The drawing under review shows one solid part. Ordinate dimensions are in mm from its lowest x, y, z. Coordinates: 2 decimals unless noted, no trailing zeros. Write each loop counter-clockwise with the first axis right and the second up, starting at its lowest first coordinate (ties: lowest second). Pieces come first, ordered by that corner, then holes.
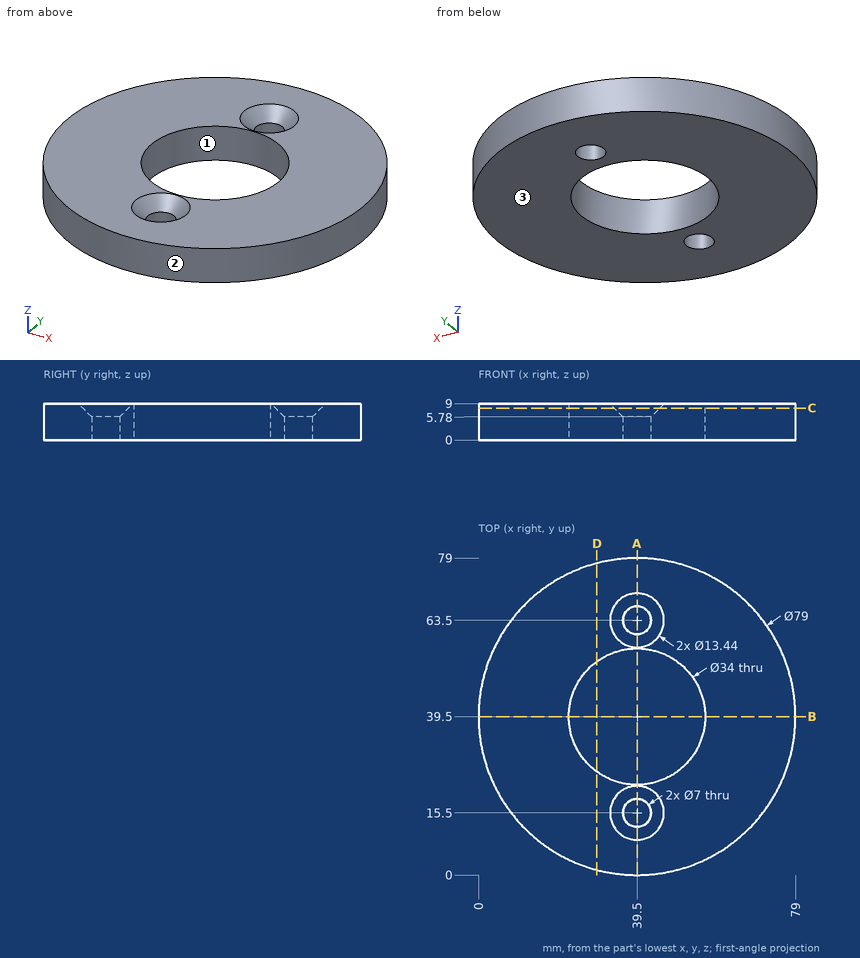
Q1. Add section B-B (y = 39.5). State the section outline as (x, z) points, then the cut area to 3 significant figures.
Ans:
outline: (0, 0) - (22.5, 0) - (22.5, 9) - (0, 9) - close; (56.5, 0) - (79, 0) - (79, 9) - (56.5, 9) - close
area: 405 mm2
Q2. Clearance check with flat-ended pins moving along their axes: pin 1 Ø4 at (y, z) = (57, 7) entering from +X; pin 2 Ø3 at (y, z) = (20.5, 7) entering from +X; pin 3 Ø2 at (x, z) = (59, 7) entering from +Y. State where each tip first meets the part, or that it passes through.
Ans:
pin 1: stops at x = 75.83
pin 2: stops at x = 74.91
pin 3: stops at y = 74.4
Q3. Add section D-D (x = 29.5). State the section outline as (y, z) points.
Ans:
outline: (1.29, 0) - (25.75, 0) - (25.75, 9) - (1.29, 9) - close; (53.25, 0) - (77.71, 0) - (77.71, 9) - (53.25, 9) - close
Q4. Draft analysis for pull direction X (two halves, no side actions). For the marked faces 1, 2 and 3, state which applies: +X half, -X half, draft (parallel to the pull), parting line (faces both ways), or undercut.
Ans:
face 1: undercut
face 2: parting line
face 3: draft
Q5. Add section C-C (z = 8). State the section outline as (x, y) points, then the cut area to 3 significant figures.
Ans:
outline: circle Ø79 at (39.5, 39.5); hole circle Ø34 at (39.5, 39.5); hole circle Ø11.44 at (39.5, 15.5); hole circle Ø11.44 at (39.5, 63.5)
area: 3,790 mm2
Q6. Add section A-A (x = 39.5). State the section outline as (y, z) points.
Ans:
outline: (0, 0) - (12, 0) - (12, 5.78) - (8.78, 9) - (0, 9) - close; (19, 0) - (22.5, 0) - (22.5, 9) - (22.22, 9) - (19, 5.78) - close; (56.5, 0) - (60, 0) - (60, 5.78) - (56.78, 9) - (56.5, 9) - close; (67, 0) - (79, 0) - (79, 9) - (70.22, 9) - (67, 5.78) - close
Q7. For probe 1 along Y at (x, z) = (39.5, 2.5); probe 2 along Y at (x, z) = (39.5, 6.25); probe 3 along X at (y, z) = (15.5, 2.45), list the stretches that pass through material, from the lowest coordinate up.
Ans:
probe 1: y = 0 to 12, 19 to 22.5, 56.5 to 60, 67 to 79
probe 2: y = 0 to 11.53, 19.47 to 22.5, 56.5 to 59.53, 67.47 to 79
probe 3: x = 8.13 to 36, 43 to 70.87
